The model under review builds one solid part; all positions refer to its coordinate system, in mm. Coordinates: 2 decimals unless noted, no trailing zeros. Write each loop counter-clockwise with the first axis right and the second up, starting at its lowest first coordinate (ties: lowest second). Pieces come first, ordered by that corner, then holes. Notation, with made-up numbers: (75.25, 44) -> (99.25, 44) arc R14 ccw to (99.25, 61) -> close; hole circle Ø9 at (70, 61). An arc over 180 degrees is marked (long way). Write each question's results on one line, items separated by ' | '.
```python
from build123d import *

# Parameters (mm, degrees)
SKETCH1_W           = 80
SKETCH1_H           = 15
BOSS_EXTRUDE1_DEPTH = 6.35
SKETCH2_R           = 3.25
CUT_EXTRUDE1_DEPTH  = 42.189470742
FILLET1_RADIUS      = 7.5
FILLET1_LENGTH      = 6.35
FILLET2_RADIUS      = 7.5
FILLET2_LENGTH      = 6.35


with BuildPart() as part:
    # Sketch1 → Boss-Extrude1 (new body)
    with BuildSketch(Plane(origin=(0, 0, 0), x_dir=(1, 0, 0), z_dir=(0, 1, 0))):
        Rectangle(SKETCH1_W, SKETCH1_H)
    extrude(amount=BOSS_EXTRUDE1_DEPTH)

    # Sketch2 → Cut-Extrude1 (cut, through all)
    with BuildSketch(Plane(origin=(0, 6.35, 0), x_dir=(1, 0, 0), z_dir=(0, 1, 0))):
        with Locations(Location((-30, 0, 0), (0, 0, 270))):
            Circle(SKETCH2_R)
        with Locations(Location((30, 0, 0), (0, 0, 270))):
            Circle(SKETCH2_R)
    extrude(amount=-CUT_EXTRUDE1_DEPTH, mode=Mode.SUBTRACT)

    # Fillet1: full round fillet: the end face becomes a half cylinder, R = half its width
    fillet1_face = Plane((-40, 3.175, 0), x_dir=(0, 1, 0), z_dir=(-1, 0, 0))  # on the end face: x along it, z out of the body
    fillet1_slab = fillet1_face.offset(-FILLET1_RADIUS / 2) * Box(FILLET1_LENGTH, 2 * FILLET1_RADIUS, FILLET1_RADIUS, mode=Mode.PRIVATE)  # the body's end, R deep
    fillet1_round = Plane((-32.5, 3.175, 0), x_dir=(-1, 0, 0), z_dir=(0, 1, 0)) * Cylinder(FILLET1_RADIUS, FILLET1_LENGTH, mode=Mode.PRIVATE)  # its axis R under the face
    add(fillet1_slab - fillet1_round, mode=Mode.SUBTRACT)

    # Fillet2: full round fillet: the end face becomes a half cylinder, R = half its width
    fillet2_face = Plane((40, 3.175, 0), x_dir=(0, -1, 0), z_dir=(1, 0, 0))  # on the end face: x along it, z out of the body
    fillet2_slab = fillet2_face.offset(-FILLET2_RADIUS / 2) * Box(FILLET2_LENGTH, 2 * FILLET2_RADIUS, FILLET2_RADIUS, mode=Mode.PRIVATE)  # the body's end, R deep
    fillet2_round = Plane((32.5, 3.175, 0), x_dir=(1, 0, 0), z_dir=(0, -1, 0)) * Cylinder(FILLET2_RADIUS, FILLET2_LENGTH, mode=Mode.PRIVATE)  # its axis R under the face
    add(fillet2_slab - fillet2_round, mode=Mode.SUBTRACT)


solid = part.part
```
Q1. For line 1 (X direction, y = 1.75, z = 0); line 2 (X direction, y = 0.75, z = 2); line 3 (Z direction, x = -27.5, y = 3.5), list the stretches that pass through material, from the lowest coordinate up. Write a range as from..to.
Solution:
line 1: -40..-33.25, -26.75..26.75, 33.25..40 | line 2: -39.73..-32.56, -27.44..27.44, 32.56..39.73 | line 3: -7.5..-2.08, 2.08..7.5
Q2. Add section C-C (y = 3.25). Write out the cut boundary in (x, z).
Solution:
outline: (-32.5, -7.5) -> (32.5, -7.5) arc R7.5 ccw to (32.5, 7.5) -> (-32.5, 7.5) arc R7.5 ccw to start; hole circle Ø6.5 at (-30, 0); hole circle Ø6.5 at (30, 0)
Q3. Clearance check with a flat-ended pin moving along its axis: P1, Ø5, axis at x = -30, z = 0, coming from the +Y side. State where the tip first meets the part, or that it passes through.
Solution:
P1: through
Q4. Add section A-A (x = -30). Write out the cut boundary in (y, z).
Solution:
outline: (0, -7.5) -> (6.35, -7.5) -> (6.35, -3.25) -> (0, -3.25) -> close; (0, 3.25) -> (6.35, 3.25) -> (6.35, 7.5) -> (0, 7.5) -> close
Q5. Add section B-B (z = 0). Write out the cut boundary in (x, y), plus the area to 3 significant figures.
Solution:
outline: (-40, 0) -> (-33.25, 0) -> (-33.25, 6.35) -> (-40, 6.35) -> close; (-26.75, 0) -> (26.75, 0) -> (26.75, 6.35) -> (-26.75, 6.35) -> close; (33.25, 0) -> (40, 0) -> (40, 6.35) -> (33.25, 6.35) -> close | area: 425 mm²
Q6. Draft analysis for pull direction X (two halves, no side actions). For faces 1 (the flat face through (0, 3, -7.5)), 2 (the cylindrical face through (-33.173, 3.219, -0.705)), 3 (the cylindrical face through (40, 3, 0)), state which applies: pulls with the +X half, pulls with the -X half, needs draft (parallel to the pull), parting line crosses it, or undercut.
Solution:
face 1: needs draft | face 2: undercut | face 3: pulls with the +X half
Q7. Add section D-D (z = 4.5). Write out the cut boundary in (x, y), plus the area to 3 significant figures.
Solution:
outline: (-38.5, 0) -> (38.5, 0) -> (38.5, 6.35) -> (-38.5, 6.35) -> close | area: 489 mm²
